The model under review builds one solid part; all positions refer to its coordinate system, in mm. Face numbers are marked on the shaded views. A direction names the side the tool comes from. Give positions to 0.01 mm unless a question says otherwise; leave off trailing zeros. Loops run counter-clockwise (first coordinate to the right, second up) from the corner with the lowest first, then second, coordinate; pieces in that order, holes last. Notation, with made-up numbers: M 48,83.25 L 57,83.25 A21 ccw 57,99.25 Z; hole C 71,-34.75 d4. An arc over 180 degrees is marked long. Return JSON: item names as keys, results as strings. Group by question number.
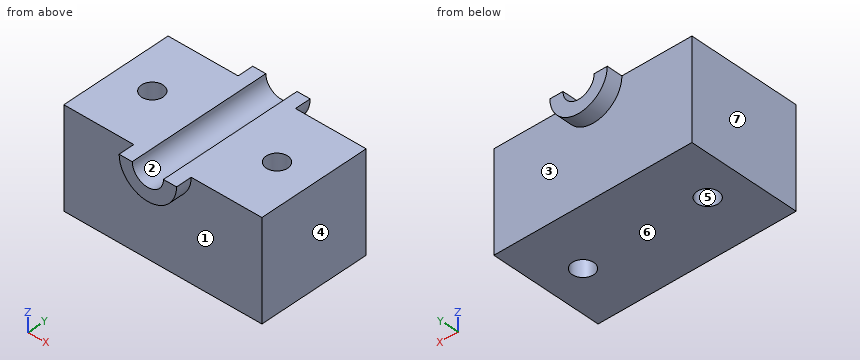
```python
from build123d import *

# Parameters (mm, degrees)
F1_DEPTH = 43.434
F2_DEPTH = 55.626
F3_R     = 8.3189115378
F4_DEPTH = 76.3916911016


# Not quite as in the source:
# - a pattern or mirror of a feature is missing from the dataset's text; its kind, count and spacing are read off the source's solid


with BuildPart() as f1:
    # F0 (on Front) → F1 (new body, symmetric)
    with BuildSketch(Plane.XZ):
        with BuildLine():
            ThreePointArc((22.2132560443, 0), (0, -22.2132560443), (-22.2132560443, 0))
            Line((-22.2132560443, 0), (-76.3906985521, 0))
            Line((-76.3906985521, 0), (-76.3906985521, -76.3906911016))
            Line((-76.3906985521, -76.3906911016), (76.9618302584, -76.3906911016))
            Line((76.9618302584, -76.3906911016), (76.9618302584, 0))
            Line((76.9618302584, 0), (22.2132560443, 0))
        make_face()
    extrude(amount=F1_DEPTH, both=True)

    # F0 (on Front) → F2 (join, symmetric)
    with BuildSketch(Plane.XZ):
        with BuildLine():
            ThreePointArc((12.0770555024, 0), (0, -12.0770555024), (-12.0770555024, 0))
            Line((-12.0770555024, 0), (-22.2132560443, 0))
            ThreePointArc((-22.2132560443, 0), (0, -22.2132560443), (22.2132560443, 0))
            Line((22.2132560443, 0), (12.0770555024, 0))
        make_face()
    extrude(amount=F2_DEPTH, both=True)

    # F3 (on face) → F4 (cut, through all)
    with BuildSketch(Plane.XY):
        with Locations((48.2908003032, 0)):
            Circle(F3_R)
    f4 = extrude(amount=-F4_DEPTH, mode=Mode.SUBTRACT)

    # F4_copies: F4 across plane
    add(f4.mirror(Plane(origin=(0, 0, 0), x_dir=(0, 0, -1), z_dir=(-1, 0, 0))), mode=Mode.SUBTRACT)


solid = f1.part
```
(1) For the marked faces 1, 2 and 3, list the 3-axis set-ups (+Z, -Z, +X, -X, +Y, -Y) from which the entire face can be reached by the end or side of a thin tool; tool diameter is ignored.
(2) Add section D-D (z = -65.5). Write out the cut boundary in (x, y), and give its area (3 significant figures).
(3) Mouldability with a two-part tool opening along X and no side actions: class the marked faces 4, 5, 6 and 7 as released by +X, released by -X, zero draft, split by the parting line, or undercut.
(4) Add section C-C (x = 0). Write out the cut boundary in (y, z).
(5) Add section B-B (y = -3.5). Write out the cut boundary in (x, z).
(6) For pin 1 (2 mm diameter, centred on x = 31.5, z = -26, fed in from +Y); pin 2 (23 mm diameter, centred on x = -21, z = -32, fed in from -Y); pin 3 (10 mm diameter, centred on x = 5, y = 25, fed in from +Z); pin 4 (10 mm diameter, centred on x = 48.29, y = 0, fed in from -Z), all flat-tipped, find the tip position at first contact; note any pin that passes through.
(7) For probe 1 along Y at (x, z) = (-47.5, -61); probe 2 along Y at (x, z) = (-7.5, -34); probe 3 along X at (y, z) = (23.5, -2.5), list the stretches that pass through material, from the lowest coordinate up.
(8) Add section A-A (z = -7.5). Write out the cut boundary in (x, y).
Verdict:
{
 "1": {"face 1": "-Z, -Y", "face 2": "+Z, +Y, -Y", "face 3": "-Z, +Y"},
 "2": {"outline": "M -76.39,-43.43 L 76.96,-43.43 L 76.96,43.43 L -76.39,43.43 Z; hole C -48.29,0 d16.64; hole C 48.29,0 d16.64", "area": "12,900 mm²"},
 "3": {"face 4": "released by +X", "face 5": "undercut", "face 6": "zero draft", "face 7": "released by -X"},
 "4": {"outline": "M -55.63,-22.21 L -43.43,-22.21 L -43.43,-76.39 L 43.43,-76.39 L 43.43,-22.21 L 55.63,-22.21 L 55.63,-12.08 L -55.63,-12.08 Z"},
 "5": {"outline": "M -76.39,-76.39 L -55.84,-76.39 L -55.84,0 L -76.39,0 Z; M -40.74,-76.39 L 40.74,-76.39 L 40.74,0 L 12.08,0 A12.08 cw -12.08,0 L -40.74,0 Z; M 55.84,-76.39 L 76.96,-76.39 L 76.96,0 L 55.84,0 Z"},
 "6": {"pin 1": "stops at y = 43.43", "pin 2": "stops at y = -43.43", "pin 3": "stops at z = -6.77", "pin 4": "passes through"},
 "7": {"probe 1": "y = -43.43 to -8.28, 8.28 to 43.43", "probe 2": "y = -43.43 to 43.43", "probe 3": "x = -76.39 to -11.82, 11.82 to 76.96"},
 "8": {"outline": "M -76.39,-43.43 L -20.91,-43.43 L -20.91,-55.63 L -9.47,-55.63 L -9.47,55.63 L -20.91,55.63 L -20.91,43.43 L -76.39,43.43 Z; M 9.47,-55.63 L 20.91,-55.63 L 20.91,-43.43 L 76.96,-43.43 L 76.96,43.43 L 20.91,43.43 L 20.91,55.63 L 9.47,55.63 Z; hole C -48.29,0 d16.64; hole C 48.29,0 d16.64"}
}
